from build123d import *

# Parameters (mm, degrees)
F0_W     = 9.525
F0_H     = 25.4
F0_W_2   = 25.4
F0_H_2   = 9.525
F1_DEPTH = 6.35
F2_DEPTH = 101.6


with BuildPart() as f1:
    # F0 (on Front) → F1 (new body)
    with BuildSketch(Plane.XZ):
        with Locations((20.6375, 0)):
            Rectangle(F0_W, F0_H)
        Polygon((12.7, -12.7), (15.875, -12.7), (15.875, 12.7), (12.7, 12.7), (12.7, 3.175), (12.7, -3.175), align=None)
        with Locations((0, -7.9375)):
            Rectangle(F0_W_2, F0_H_2)
        Polygon((-15.875, -12.7), (-12.7, -12.7), (-12.7, -3.175), (-12.7, 3.175), (-12.7, 12.7), (-15.875, 12.7), align=None)
        with Locations((0, 7.9375)):
            Rectangle(F0_W_2, F0_H_2)
        with Locations((-20.6375, 0)):
            Rectangle(F0_W, F0_H)
    extrude(amount=F1_DEPTH)

    # F0 (on Front) → F2 (join)
    with BuildSketch(Plane.XZ):
        with Locations((20.6375, 0)):
            Rectangle(F0_W, F0_H)
        with Locations((-20.6375, 0)):
            Rectangle(F0_W, F0_H)
    extrude(amount=F2_DEPTH)


solid = f1.part
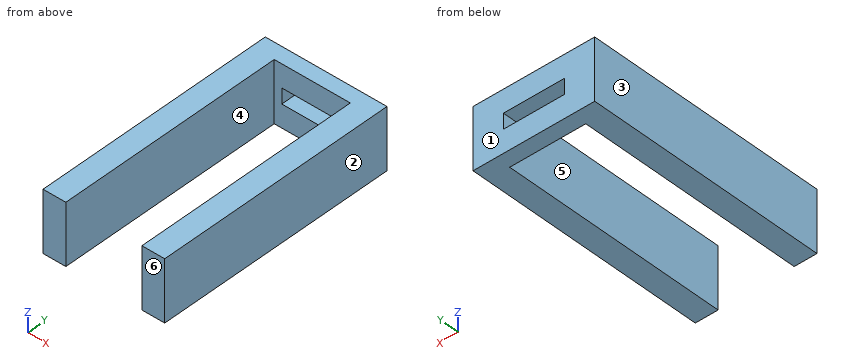
Geometry: final body of the model. Coordinates: model frame, mm. Face numbers are marked on the shaded views. A direction names the side the tool comes from. Give positions to 0.01 mm unless a question says otherwise; leave off trailing zeros. Write each loop counter-clockwise with the first axis right and the second up, starting at its lowest first coordinate (ties: lowest second). Pieces come first, ordered by that corner, then holes.
(1) Cut plane A-A, the plane z = -0.25. Return loops of the section in (x, y) (3 decimals).
(2) Mould query, pull axis X, two halves, no side actions, for the marked faces 1, 2, 3 and 4. Classes: released by +X, released by -X, zero draft, split by the parting line, or undercut.
(3) Cut plane B-B, the plane y = -87. Return loops of the section in (x, z) (3 decimals), then the cut area to 3 significant figures.
(4) Access query for the marked faces 5 and 6. Directions: +Z, -Z, +X, -X, +Y, -Y. A direction counts if a zero-diameter tool reaches every point of the face in a straight line with its end or side. Return the directions, or none.
(5) First-contact query: P1, Ø7.5, axis at x = 5, z = 3, coming from the -Y side. Flat tip, straight axial feed; report the tip coordinate or a pass-through.
(6) Ray query, line 1 (X direction, y = -41, z = -9) (3 decimals); line 2 (Y direction, x = -13, z = 9). Return the intervals inside material, ascending.
(7) Cut plane C-C, the plane x = -1. Return loops of the section in (y, z) (3 decimals).
(8) Cut plane D-D, the plane z = -10.5. Return loops of the section in (x, y) (3 decimals).
Values follow:
1. outline: (-25.4, -101.6) - (-15.875, -101.6) - (-15.875, -6.35) - (-12.7, -6.35) - (-12.7, 0) - (-25.4, 0) - close; (12.7, -6.35) - (15.875, -6.35) - (15.875, -101.6) - (25.4, -101.6) - (25.4, 0) - (12.7, 0) - close
2. face 1: zero draft
2. face 2: released by +X
2. face 3: released by -X
2. face 4: undercut
3. outline: (-25.4, -12.7) - (-15.875, -12.7) - (-15.875, 12.7) - (-25.4, 12.7) - close; (15.875, -12.7) - (25.4, -12.7) - (25.4, 12.7) - (15.875, 12.7) - close
3. area: 484 mm2
4. face 5: +Z, -Z, -Y
4. face 6: +Z, -Z, +X, -X, -Y
5. P1: stops at y = -6.35
6. line 1: x = -25.4 to -15.875, 15.875 to 25.4
6. line 2: y = -6.35 to 0
7. outline: (-6.35, -12.7) - (0, -12.7) - (0, -3.175) - (-6.35, -3.175) - close; (-6.35, 3.175) - (0, 3.175) - (0, 12.7) - (-6.35, 12.7) - close
8. outline: (-25.4, -101.6) - (-15.875, -101.6) - (-15.875, -6.35) - (15.875, -6.35) - (15.875, -101.6) - (25.4, -101.6) - (25.4, 0) - (-25.4, 0) - close
